Source: CAD feature listing. Evaluate the final solid. Frame: model axes, mm. Face numbers are marked on the shaded views. Coordinates: 2 decimals unless noted, no trailing zeros. Loops run counter-clockwise (first coordinate to the right, second up) from the corner with the lowest first, then second, coordinate; pieces in that order, holes last. Notation, with made-up numbers: (-33, 8.5) -> (-10, 8.5) arc R13 ccw to (-10, 20.5) -> close; hole circle Ø7 at (19, -36.5). An arc over 180 degrees is marked (long way). Answer as CSV lines item,"result".
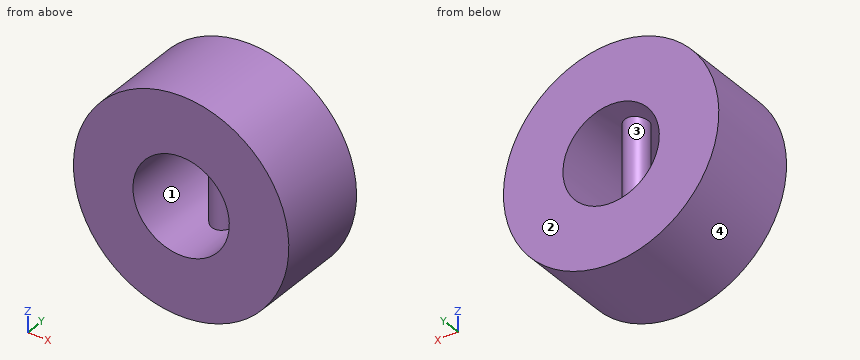
from build123d import *

# Parameters (mm, degrees)
SKETCH1_R               = 56.764595508
BOSS_EXTRUDE1_DEPTH     = 25.4
CUT_EXTRUDE1_DEPTH      = 85.199754194
CUT_EXTRUDE1_DEPTH_BACK = 85.199754194
SKETCH3_R               = 25.4
SKETCH4_W               = 12.7
SKETCH4_H               = 50.8
BOSS_EXTRUDE2_DEPTH     = 12.7
FILLET1_R               = 6.35


with BuildPart() as part:
    # Sketch1 → Boss-Extrude1 (new, symmetric)
    with BuildSketch(Plane(origin=(0, 0, 0), x_dir=(1, 0, 0), z_dir=(0, 1, 0))):
        with Locations(Location((0, 0, 0), (0, 0, 270))):
            Circle(SKETCH1_R)
    extrude(amount=BOSS_EXTRUDE1_DEPTH, both=True)

    # Sketch3 → Cut-Extrude1 (cut, two sides: drawn at the far end of the back side and taken through both)
    with BuildSketch(Plane(origin=(0, 0, 0), x_dir=(1, 0, 0), z_dir=(0, 1, 0)).offset(-CUT_EXTRUDE1_DEPTH_BACK)):
        with Locations(Location((0, 0, 0), (0, 0, 270))):
            Circle(SKETCH3_R)
    extrude(amount=CUT_EXTRUDE1_DEPTH + CUT_EXTRUDE1_DEPTH_BACK, mode=Mode.SUBTRACT)

    # Sketch4 → Boss-Extrude2 (add)
    with BuildSketch(Plane(origin=(0, 0, 0), x_dir=(1, 0, 0), z_dir=(0, 1, 0))):
        Rectangle(SKETCH4_W, SKETCH4_H)
    extrude(amount=BOSS_EXTRUDE2_DEPTH)

    # Fillet1
    # the kernel refuses this fillet: 6.35 mm, written as the material it takes off along each edge
    with BuildSketch(Plane(origin=(-6.35, 0, 40.468444248), x_dir=(0, 1, 0), z_dir=(0, 0, -1))) as fillet1_piece_1_section:
        with BuildLine():
            CenterArc((FILLET1_R, FILLET1_R), FILLET1_R, 180, 90)
            Line((0, FILLET1_R), (0, 0))
            Line((0, 0), (FILLET1_R, 0))
        make_face()
    fillet1_piece_1 = extrude(amount=80.936888497, mode=Mode.PRIVATE)
    fillet1_piece_1 = fillet1_piece_1 & Plane(origin=(0, 1.429605244, 0), x_dir=(0, 0, 1), z_dir=(0, 1, 0)) * Cylinder(25.4, 188, mode=Mode.PRIVATE)
    with BuildSketch(Plane(origin=(-6.35, 12.7, 40.468444248), x_dir=(1, 0, 0), z_dir=(0, 0, -1))) as fillet1_piece_2_section:
        with BuildLine():
            CenterArc((FILLET1_R, FILLET1_R), FILLET1_R, 180, 90)
            Line((0, FILLET1_R), (0, 0))
            Line((0, 0), (FILLET1_R, 0))
        make_face()
    fillet1_piece_2 = extrude(amount=80.936888497, mode=Mode.PRIVATE)
    fillet1_piece_2 = fillet1_piece_2 & Plane(origin=(0, 11.270396349, 0), x_dir=(0, 0, 1), z_dir=(0, 1, 0)) * Cylinder(25.4, 188, mode=Mode.PRIVATE)
    with BuildSketch(Plane(origin=(6.35, 0, -40.468444248), x_dir=(0, 1, 0), z_dir=(0, 0, 1))) as fillet1_piece_3_section:
        with BuildLine():
            CenterArc((FILLET1_R, FILLET1_R), FILLET1_R, 180, 90)
            Line((0, FILLET1_R), (0, 0))
            Line((0, 0), (FILLET1_R, 0))
        make_face()
    fillet1_piece_3 = extrude(amount=80.936888497, mode=Mode.PRIVATE)
    fillet1_piece_3 = fillet1_piece_3 & Plane(origin=(0, 1.429603632, 0), x_dir=(0, 0, 1), z_dir=(0, 1, 0)) * Cylinder(25.4, 188, mode=Mode.PRIVATE)
    with BuildSketch(Plane(origin=(6.35, 12.7, -40.468444248), x_dir=(0, -1, 0), z_dir=(0, 0, 1))) as fillet1_piece_4_section:
        with BuildLine():
            CenterArc((FILLET1_R, -FILLET1_R), FILLET1_R, 90, 90)
            Line((0, -FILLET1_R), (0, 0))
            Line((0, 0), (FILLET1_R, 0))
        make_face()
    fillet1_piece_4 = extrude(amount=80.936888497, mode=Mode.PRIVATE)
    fillet1_piece_4 = fillet1_piece_4 & Plane(origin=(0, 11.270396368, 0), x_dir=(0, 0, 1), z_dir=(0, 1, 0)) * Cylinder(25.4, 188, mode=Mode.PRIVATE)
    add([fillet1_piece_1, fillet1_piece_2, fillet1_piece_3, fillet1_piece_4], mode=Mode.SUBTRACT)


solid = part.part
(1) Draft query along Z for the marked faces 1, 2, 3 and 4. Return one class per face: released by +Z, released by -Z, zero draft, split by the parting line, or undercut.
Computed values:
face 1,"undercut"
face 2,"zero draft"
face 3,"undercut"
face 4,"split by the parting line"
(2) Cut plane A-A (z = 0). Return the cut outline in (x, y).
Computed values:
outline,"(-56.76, -25.4) -> (-25.4, -25.4) -> (-25.4, 25.4) -> (-56.76, 25.4) -> close; circle Ø12.7 at (0, 6.35); (25.4, -25.4) -> (56.76, -25.4) -> (56.76, 25.4) -> (25.4, 25.4) -> close"
(3) Material intervals for L1, parallel to X at y = -3, z = 0; L2, parallel to X at y = 8.5, z = 15; L3, parallel to X at y = 12, z = 4.5, sorted ascending. Write a range as [from, to].
Computed values:
L1,"[-56.76, -25.4], [25.4, 56.76]"
L2,"[-54.75, -20.5], [-5.97, 5.97], [20.5, 54.75]"
L3,"[-56.59, -25], [-2.9, 2.9], [25, 56.59]"
(4) Cut plane D-D (y = 6.35). Return the cut outline in (x, z), then the cut area to 3 significant figures.
Computed values:
outline,"circle Ø113.53 at (0, 0); hole (-6.35, -24.59) -> (-6.35, 24.59) arc R25.4 ccw to start; hole (6.35, -24.59) arc R25.4 ccw to (6.35, 24.59) -> close"
area,"8,730 mm^2"
(5) Cut plane C-C (x = 13). Return the cut outline in (y, z).
Computed values:
outline,"(-25.4, -55.26) -> (25.4, -55.26) -> (25.4, -21.82) -> (-25.4, -21.82) -> close; (-25.4, 21.82) -> (25.4, 21.82) -> (25.4, 55.26) -> (-25.4, 55.26) -> close"
(6) Pin query (flat end, axial travel): pin 1 Ø3 at (x, y) = (16.5, -9) entering from +Z; pin 2 Ø4 at (x, y) = (-44.5, 4.5) entering from +Z; pin 3 Ø8 at (x, z) = (-7, 14.5) entering from +Y. Return the tip coordinate at first contact, or that it passes through.
Computed values:
pin 1,"z = 54.75"
pin 2,"z = 37.63"
pin 3,"y = 11.95"
(7) Cut plane B-B (x = 0). Return the cut outline in (y, z), then the cut area to 3 significant figures.
Computed values:
outline,"(-25.4, -56.76) -> (25.4, -56.76) -> (25.4, -25.4) -> (12.7, -25.4) -> (12.7, 25.4) -> (25.4, 25.4) -> (25.4, 56.76) -> (-25.4, 56.76) -> (-25.4, 25.4) -> (0, 25.4) -> (0, -25.4) -> (-25.4, -25.4) -> close"
area,"3,830 mm^2"
